For this review, take the finished solid that the model builds, in its own axes (mm). A direction names the side the tool comes from. Give positions to 0.01 mm unless a question says otherwise; leave off trailing zeros. Loops run counter-clockwise (first coordinate to the right, second up) from the corner with the lowest first, then second, coordinate; pieces in that order, holes last. Notation, with made-up numbers: (40.25, 49.25) -> (89.25, 49.25) arc R27 cw to (89.25, 82.25) -> close; hole circle Ø11 at (13, 48.25). An arc over 180 degrees is marked (long way). One line per question, with ' | ' between items. Start each with the question number.
(1) Wall thickness on probe 1 along X at (y, z) = (-1.35, 0); probe 2 along Z at (x, y) = (5.9, -0.4); probe 3 along X at (y, z) = (1.8, 9.5): over which ranges is each line inside the solid? List them lowest first.
(2) Consider section A-A (y = 0.8). Write out the cut boundary in (x, z).
(3) Tool access review of faces 5 (the flat face through (1, -2, 10)), 6 (the flat face through (-9, 0, -1)), 7 (the flat face through (-41, -1, -3)), 8 (the flat face through (2, 0, -46)), 9 (the flat face through (-45.1, -0.4, 2)): name each direction out of +Z, -Z, +X, -X, +Y, -Y from which nothing blocks a thin tool from reaching the whole face with its end or side.
(4) Consider section B-B (z = 28). Write out the cut boundary in (x, y), and give its area (3 significant figures).
(5) Draft analysis for pull direction Z (two halves, no side actions). For faces 1 (the flat face through (-2, -0.4, -45.1)), 2 (the flat face through (3, -1, -41)), 3 (the cylindrical face through (32.14, -0.028, 34.293)), 4 (the cylindrical face through (-32.887, -0.028, -33.578)), state which applies: +Z half, -Z half, draft (parallel to the pull), parting line (faces both ways), or undercut.
(6) Consider section C-C (x = 15). Write out the cut boundary in (y, z), and give its area (3 significant figures).
(7) Insertion check: P1, Ø1, axis at x = 1, z = 25, coming from the +Y side; P2, Ø2, axis at x = -44, y = 0.5, coming from the -Z side; P3, Ø2, axis at x = 6, y = -1, coming from the +Z side. Each pin has a flat end and moves straight along its axis. Give the tip position at first contact, or say it passes through.
from build123d import *

# Parameters (mm, degrees)
SKETCH1_R                     = 45
OUTER_DISK_DEPTH              = 2
ENCLOSEMENT_T                 = 2
HOOK_RELEASE_DEPTH            = 67.498120274
CIRPATTERN1_COUNT             = 2
CIRPATTERN1_ANGLE             = 90
SERVO_MOTOR_CUTOUT_DEPTH      = 67.498120274
SERVO_MOTOR_CUTOUT_DEPTH_BACK = 67.498120274
SKETCH3_R                     = 3
SKETCH3_R_2                   = 5.9
FILLET1_R                     = 1


with BuildPart() as part:
    # Sketch1 → Outer DIsk (new body)
    with BuildSketch(Plane(origin=(0, 0, 0), x_dir=(1, 0, 0), z_dir=(0, 1, 0))):
        with Locations(Location((0, 0, 0), (0, 0, 270))):
            Circle(SKETCH1_R)
    extrude(amount=OUTER_DISK_DEPTH)

    # Enclosement
    enclosement_openings = [part.faces().sort_by_distance(p)[0] for p in [
        (0, 2, 0),
    ]]
    offset(amount=ENCLOSEMENT_T, openings=enclosement_openings, kind=Kind.INTERSECTION)

    # Sketch2 → Hook Release (cut, symmetric)
    with BuildSketch(Plane(origin=(0, 0, 0), x_dir=(1, 0, 0), z_dir=(0, 1, 0))):
        Polygon((-2, 47), (-2, 41), (8, 41), (8, 43), (2, 43), (2, 47), align=None)
    hook_release = extrude(amount=HOOK_RELEASE_DEPTH, both=True, mode=Mode.SUBTRACT)

    # CirPattern1: Hook Release ×2 about axis
    cirpattern1_axis = Axis((0, 0, 0), (0, 1, 0))
    for i in range(1, CIRPATTERN1_COUNT):
        add(hook_release.rotate(cirpattern1_axis, i * CIRPATTERN1_ANGLE / (CIRPATTERN1_COUNT - 1)), mode=Mode.SUBTRACT)

    # Sketch3 → Servo Motor Cutout (cut, two sides: drawn at the far end of the back side and taken through both)
    with BuildSketch(Plane(origin=(0, 0, 0), x_dir=(1, 0, 0), z_dir=(0, 1, 0)).offset(-SERVO_MOTOR_CUTOUT_DEPTH_BACK)):
        with Locations((5.9, 0)):
            Circle(SKETCH3_R)
        Circle(SKETCH3_R_2)
    extrude(amount=SERVO_MOTOR_CUTOUT_DEPTH + SERVO_MOTOR_CUTOUT_DEPTH_BACK, mode=Mode.SUBTRACT)

    # Fillet1
    fillet1_edges = [part.edges().sort_by_distance(p)[0] for p in [
        (-41, -1, 2),
        (-41, -1, -8),
        (-43, -1, -8),
        (-43, -1, -2),
        (8, -1, -41),
        (-2, -1, -41),
        (8, -1, -43),
        (2, -1, -43),
    ]]
    fillet(fillet1_edges, radius=FILLET1_R - 0.0001)  # a hair under: the kernel refuses the full size


solid = part.part
A:
1) probe 1: x = -41 to -5.9, 8.9 to 47 | probe 2: z = -46.63 to -43, -41 to -3, 3 to 46.63 | probe 3: x = -46.03 to -43.99, 43.99 to 46.03
2) outline: (-46.96, -2) arc R47 ccw to (-2, -46.96) -> (-2, -44.96) arc R45 cw to (-44.96, -2) -> close; (-46.96, 2) -> (-44.96, 2) arc R45 cw (long way) to (2, -44.96) -> (2, -46.96) arc R47 ccw (long way) to start
3) face 5: +Z, -Z, +X, -X, -Y | face 6: +Y | face 7: +Y, -Y | face 8: -Z, +Y, -Y | face 9: -X, +Y, -Y
4) outline: (-37.75, -2) -> (37.75, -2) -> (37.75, 2) -> (35.23, 2) -> (35.23, 0) -> (-35.23, 0) -> (-35.23, 2) -> (-37.75, 2) -> close | area: 161 mm^2
5) face 1: draft | face 2: undercut | face 3: parting line | face 4: -Z half
6) outline: (-2, -44.54) -> (2, -44.54) -> (2, -42.43) -> (0, -42.43) -> (0, 42.43) -> (2, 42.43) -> (2, 44.54) -> (-2, 44.54) -> close | area: 187 mm^2
7) P1: stops at y = 0 | P2: stops at z = -18.97 | P3: stops at z = 46.73
